Could you check a few things on this drawing? It's one solid part, dimensions in mm from its lowest x, y, z. Give positions to 0.01 mm unless a question says otherwise; leave off trailing zeros. Write each loop counter-clockwise with the first axis right and the second up, starting at its lowest first coordinate (ties: lowest second). Pieces come first, ordered by that corner, then holes. Notation, with made-up numbers: M 7.25,-20.75 L 63.25,-20.75 A24 ccw 63.25,2.25 Z; hole C 26.5,46.25 d10. An arc over 180 degrees is marked long. Use CSV: the item, a comma, the result in double quotes. Start each with the question number.
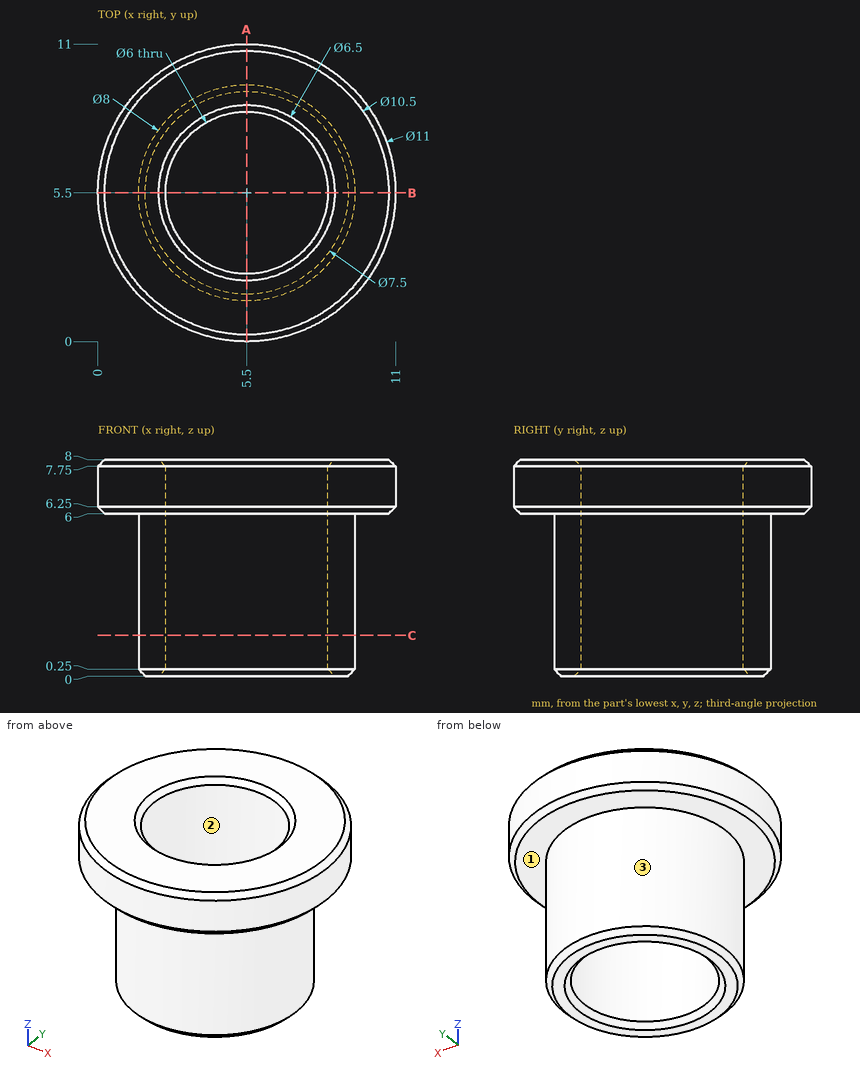
(1) Will these pins go through, and if not, where does the flat tip stop? pin 1 Ø2 at (x, z) = (10, 6.5) entering from +Y; pin 2 Ø3.5 at (x, y) = (5.5, 5.5) entering from +Z.
(2) Thinking about a two-plate mould opening in X: for the marked faces 1, 2 and 3, which applies, released by +X, released by -X, zero draft, split by the parting line, or undercut?
(3) Please list where these lines run through material, in increasing order: L1, parallel to X at y = 5.5, z = 4.25; L2, parallel to Z at x = 2.5, y = 1.75; L3, parallel to Y at x = 8, z = 7.5. Write a range as [from, to].
(4) I want a section at C-C (z = 1.5). Write out the boundary of the cut face in (x, y).
(5) I want a section at A-A (x = 5.5). Write out the boundary of the cut face in (y, z), and give its area (3 significant figures).
Geometry results:
1,pin 1,"stops at y = 9.74"
1,pin 2,"passes through"
2,face 1,"zero draft"
2,face 2,"undercut"
2,face 3,"split by the parting line"
3,L1,"x = [1.5, 2.5], [8.5, 9.5]"
3,L2,"z = [6, 8]"
3,L3,"y = [0.6, 3.84], [7.16, 10.4]"
4,outline,"C 5.5,5.5 d8; hole C 5.5,5.5 d6"
5,outline,"M 0,6.25 L 0.25,6 L 1.5,6 L 1.5,0.25 L 1.75,0 L 2.25,0 L 2.5,0.25 L 2.5,7.75 L 2.25,8 L 0.25,8 L 0,7.75 Z; M 8.5,0.25 L 8.75,0 L 9.25,0 L 9.5,0.25 L 9.5,6 L 10.75,6 L 11,6.25 L 11,7.75 L 10.75,8 L 8.75,8 L 8.5,7.75 Z"
5,area,"21.7 mm2"
